Autodesk Inventor part; units mm, degrees
ref_plane "YZ Plane" through (0, 0, 0) normal (1, 0, 0) x (0, 1, 0)
ref_plane "XZ Plane" through (0, 0, 0) normal (0, 1, 0) x (-1, 0, 0)
ref_plane "XY Plane" through (0, 0, 0) normal (0, 0, 1) x (1, 0, 0)
sketch "Sketch1" plane through (0, 0, 0) normal (0, 0, 1) x (1, 0, 0)
  line L0 (-27.4801, 0) -> (27.4801, 0) construction
  line L1 (0, -17.6656) -> (0, 17.6656) construction
  line L2 (-16.256, 12.0396) -> (16.256, 12.0396)
  line L3 (19.05, 9.2456) -> (19.05, -9.2456)
  line L4 (16.256, -12.0396) -> (-16.256, -12.0396)
  line L5 (-19.05, -9.2456) -> (-19.05, 9.2456)
  line L6 (-16.256, 9.2456) -> (-16.256, -9.2456) construction
  circle A0 centre (-16.256, 9.2456) radius 1.2192
  circle A1 centre (-16.256, -9.2456) radius 1.2192
  circle A2 centre (16.256, 0) radius 1.2192
  arc A3 (-16.256, 12.0396) -> (-19.05, 9.2456) centre (-16.256, 9.2456) ccw
  arc A4 (-19.05, -9.2456) -> (-16.256, -12.0396) centre (-16.256, -9.2456) ccw
  arc A5 (16.256, -12.0396) -> (19.05, -9.2456) centre (16.256, -9.2456) ccw
  arc A6 (19.05, 9.2456) -> (16.256, 12.0396) centre (16.256, 9.2456) ccw
  line L7 (-16.256, 9.2456) -> (-12.4968, 9.2456) construction
  line L8 (-12.4968, 6.4516) -> (-16.256, 6.4516)
  arc A7 (-16.256, 12.0396) -> (-16.256, 6.4516) centre (-16.256, 9.2456) ccw
  arc A8 (-12.4968, 6.4516) -> (-12.4968, 12.0396) centre (-12.4968, 9.2456) ccw
  line L9 (-16.256, -9.2456) -> (-12.4968, -9.2456) construction
  line L10 (-12.4968, -6.4516) -> (-16.256, -6.4516)
  arc A9 (-16.256, -6.4516) -> (-19.05, -9.2456) centre (-16.256, -9.2456) ccw
  arc A10 (-12.4968, -12.0396) -> (-12.4968, -6.4516) centre (-12.4968, -9.2456) ccw
  circle A11 centre (-11.556, 9.2456) radius 1.2192
  circle A12 centre (-11.556, -9.2456) radius 1.2192
  line L11 (-11.556, 9.2456) -> (-11.556, -9.2456) construction
  line L12 (-12.7, 5.9436) -> (-12.7, -5.9436)
  arc A13 (-12.7, 5.9436) -> (-13.208, 6.4516) centre (-13.208, 5.9436) ccw
  arc A14 (-13.208, -6.4516) -> (-12.7, -5.9436) centre (-13.208, -5.9436) ccw
  circle A15 centre (16.256, 0) radius 2.794
  point P0 (0, 0)
  point P1 (19.05, -12.0396)
  point P2 (19.05, 12.0396)
  point P3 (-19.05, -12.0396)
  point P4 (-14.3764, 9.2456)
  point P5 (-14.3764, -9.2456)
  dimension "d0" = 38.1
  dimension "d1" = 24.0792
  dimension "d2" = 18.4912
  dimension "d3" = 2.4384
  dimension "d4" = 32.512
  dimension "d7" = 3.7592
  dimension "d8" = 4.7
  dimension "d9" = 6.35
  dimension "d12" = 0.508
extrude "Extrusion1" add sketch "Sketch1" along normal blind 1.905 contours L2 A8 L8 A7 A3 | A15 | L2 A6 L3 A5 L4 A10 L10 A14 L12 A13 L8 A8 | A7 L8 A13 L12 A14 L10 A9 L5 | A9 L10 A10 L4 A4 | A11 | A12
extrude "Extrusion2" add sketch "Sketch1" along normal blind 6.985 from surface at 1.905 contours L2 A8 L8 A7 A3 | A15 | L2 A6 L3 A5 L4 A10 L10 A14 L12 A13 L8 A8 | A9 L10 A10 L4 A4
extrude "Extrusion3" add sketch "Sketch1" along normal blind 0.889 from surface at 8.89 contours L2 A8 L8 A7 A3 | A15 | A9 L10 A10 L4 A4
properties part number "Lord Microstrain 3DM-CX5 OEM"
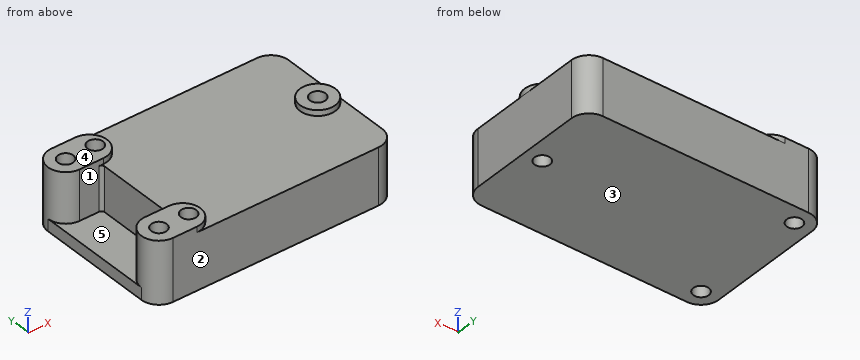
Geometry: final body of the model. Coordinates: model frame, mm. Face numbers are marked on the shaded views. A direction names the side the tool comes from. Round coordinates to 2 decimals unless told otherwise and drop trailing zeros. Order: outer loops, then holes, each group sorted by start corner. A loop starts at its lowest first (then second) coordinate and runs counter-clockwise, first axis right, second up. Notation, with made-up numbers: (71, -32) -> (97, -32) arc R30 cw to (97, 7) -> close; hole circle Ø8 at (40.25, 57.25). An arc over 180 degrees is marked (long way). Use one line per item in the form item = value.
(1) First-contact query: pin 1 Ø3 at (x, y) = (12.5, -9.5) entering from +Z; pin 2 Ø1.2 at (x, y) = (-11.5, 9) entering from +Z (3 decimals). Flat tips, straight axial feed; report the tip coordinate or a pass-through.
Results list:
pin_1 = 8.89
pin_2 = 1.905
(2) Section A-A on z = 2.75. Return loops of the section in (x, y).
Results list:
outline = (-16.26, -12.04) -> (16.26, -12.04) arc R2.79 ccw to (19.05, -9.25) -> (19.05, 9.25) arc R2.79 ccw to (16.26, 12.04) -> (-16.26, 12.04) arc R2.79 ccw to (-16.26, 6.45) -> (-13.21, 6.45) arc R0.51 cw to (-12.7, 5.94) -> (-12.7, -5.94) arc R0.51 cw to (-13.21, -6.45) -> (-16.26, -6.45) arc R2.79 ccw to start; hole circle Ø2.44 at (-16.26, -9.25); hole circle Ø2.44 at (-16.26, 9.25); hole circle Ø2.44 at (-11.56, -9.25); hole circle Ø2.44 at (-11.56, 9.25); hole circle Ø2.44 at (16.26, 0)
(3) Section B-B on y = -5.5. Return loops of the section in (x, z) (3 decimals), and give its area (3 significant figures).
Results list:
outline = (-19.05, 0) -> (19.05, 0) -> (19.05, 8.89) -> (-12.7, 8.89) -> (-12.7, 1.905) -> (-19.05, 1.905) -> close
area = 294 mm^2
(4) Section C-C on x = -7. Return loops of the section in (y, z), and give its area (3 significant figures).
Results list:
outline = (-12.04, 0) -> (12.04, 0) -> (12.04, 8.89) -> (-12.04, 8.89) -> close
area = 214 mm^2
(5) Ray query, probe 1 along Y at (x, z) = (-14, 5); probe 2 along Y at (x, z) = (-17, 1.75); probe 3 along Y at (x, z) = (-15.5, 6.75). Return the intervals inside material, ascending. Write a range as [from, to].
Results list:
probe_1 = [-12.04, -6.45], [6.45, 12.04]
probe_2 = [-11.94, -10.21], [-8.28, 8.28], [10.21, 11.94]
probe_3 = [-12.04, -10.2], [-8.29, -6.45], [6.45, 8.29], [10.2, 12.04]
(6) Access query for the marked faces 4 and 5. Directions: +Z, -Z, +X, -X, +Y, -Y. A direction counts if a zero-diameter tool reaches every point of the face in a straight line with its end or side. Return the directions, or none.
Results list:
face_4 = +Z, +X, -X, +Y, -Y
face_5 = +Z, -X
(7) Draft query along Y for the marked faces 1, 2 and 3. Return one class per face: pulls with the +Y half, pulls with the -Y half, needs draft (parallel to the pull), parting line crosses it, or undercut.
Results list:
face_1 = undercut
face_2 = pulls with the -Y half
face_3 = needs draft
